```python
from build123d import *

# Parameters (mm, degrees)
F0_W     = 50
F0_H     = 15
F0_R     = 5
F1_DEPTH = 10
F2_R     = 4.5
F3_DEPTH = 10


with BuildPart() as f1:
    # F0 (on Top) → F1 (new body)
    with BuildSketch(Plane.XY):
        Rectangle(F0_W, F0_H)
        with Locations((15, 0)):
            Circle(F0_R, mode=Mode.SUBTRACT)
    extrude(amount=F1_DEPTH)

    # F2 (on face) → F3 (join)
    with BuildSketch(Plane.XY.offset(10)):
        with Locations((-15, 0)):
            Circle(F2_R)
    extrude(amount=F3_DEPTH)


solid = f1.part
```
Geometry check sheet. Reference: the model listing, model coordinates, mm. A direction names the side the tool comes from. Coordinates: 2 decimals unless noted, no trailing zeros. Write each loop counter-clockwise with the first axis right and the second up, starting at its lowest first coordinate (ties: lowest second). Pieces come first, ordered by that corner, then holes. Notation, with made-up numbers: M -9.75,67.25 L 28.25,67.25 A10 ccw 28.25,74.25 Z; hole C 41,86 d10. An arc over 180 degrees is marked long. One line per item, written item: value. Start each with the question number.
(1) Release check for a two-part mould opening along Y. For faces 3 (the face through (0, -7.5, 5)), 4 (the face through (19.77, 1.5, 4.93)), 5 (the face through (-25, 0, 5)), 6 (the face through (0, 7.5, 5)) record: released by +Y, released by -Y, zero draft, split by the parting line, or undercut.
(2) Scan lines: line 1 along Y through (x, z) = (15, 5); line 2 along Z through (x, y) = (-22, 1); line 3 along X through (y, z) = (-4.5, 3.25). Record each from-to range of solid material in increasing order. Write a range as [from, to].
(3) Sectioned sample at D-D, the plane x = -15. Enter the section's corners in (y, z).
(4) Sectioned sample at A-A, the plane y = 0. Enter the section's corners in (x, z).
(5) Sectioned sample at B-B, the plane x = 15. Enter the section's corners in (y, z), and give its area (3 significant figures).
(6) Depth check by flat-ended pin: pin 1 (2 mm diameter, centred on x = 18.5, y = -2, fed in from +Z); pin 2 (1 mm diameter, centred on y = 6, z = 16, fed in from -X); pin 3 (2 mm diameter, centred on x = -2, y = -1, fed in from -Z). Enter the tip coordinate at first touch or a pass-through.
(7) Sectioned sample at C-C, the plane z = 5.75. Enter the section's corners in (x, y).
(8) Tool access check on faces 1 (the face through (0, 0, 0)), 2 (the face through (-19.496, 0.198, 14.93)). Record the directions out of +Z, -Z, +X, -X, +Y, -Y that give a thin tool (end or side, any length) a straight path to the whole face; none if there is none.
Filled sheet:
1. face 3: released by -Y
1. face 4: undercut
1. face 5: zero draft
1. face 6: released by +Y
2. line 1: [-7.5, -5], [5, 7.5]
2. line 2: [0, 10]
2. line 3: [-25, 12.82], [17.18, 25]
3. outline: M -7.5,0 L 7.5,0 L 7.5,10 L 4.5,10 L 4.5,20 L -4.5,20 L -4.5,10 L -7.5,10 Z
4. outline: M -25,0 L 10,0 L 10,10 L -10.5,10 L -10.5,20 L -19.5,20 L -19.5,10 L -25,10 Z; M 20,0 L 25,0 L 25,10 L 20,10 Z
5. outline: M -7.5,0 L -5,0 L -5,10 L -7.5,10 Z; M 5,0 L 7.5,0 L 7.5,10 L 5,10 Z
5. area: 50.0 mm²
6. pin 1: z = 10
6. pin 2: through
6. pin 3: z = 0
7. outline: M -25,-7.5 L 25,-7.5 L 25,7.5 L -25,7.5 Z; hole C 15,0 d10
8. face 1: -Z, +X, -X, +Y, -Y
8. face 2: +Z
